from build123d import *

# Parameters (mm, degrees)
CROQUIS1_R              = 10
SALIENTE_EXTRUIR1_DEPTH = 5


with BuildPart() as part:
    # Croquis1 → Saliente-Extruir1 (new body, symmetric)
    with BuildSketch(Plane.XY):
        with BuildLine():
            Line((-55, 15), (55, 15))
            ThreePointArc((55, 15), (62.071067812, 12.071067812), (65, 5))
            Line((65, 5), (65, -5))
            ThreePointArc((65, -5), (62.071067812, -12.071067812), (55, -15))
            Line((55, -15), (-55, -15))
            ThreePointArc((-55, -15), (-62.071067812, -12.071067812), (-65, -5))
            Line((-65, -5), (-65, 5))
            ThreePointArc((-65, 5), (-62.071067812, 12.071067812), (-55, 15))
        make_face()
        with Locations((-50, 0)):
            Circle(CROQUIS1_R, mode=Mode.SUBTRACT)
        with Locations((50, 0)):
            Circle(CROQUIS1_R, mode=Mode.SUBTRACT)
    extrude(amount=SALIENTE_EXTRUIR1_DEPTH, both=True)


solid = part.part
Design review of the part built by this model. Coordinates are the model's own, in mm. Round coordinates to 2 decimals unless told otherwise and drop trailing zeros. Write each loop counter-clockwise with the first axis right and the second up, starting at its lowest first coordinate (ties: lowest second). Pieces come first, ordered by that corner, then holes. Notation, with made-up numbers: M -5.75,65.25 L 4.25,65.25 A26 cw 4.25,88.25 Z; hole C -31.5,-20 d7. An arc over 180 degrees is marked long. One line per item, written item: value. Start each with the question number.
1. Take a section at B-B on x = 50. State the section outline as (y, z) points.
2. Take a section at D-D on x = -50.5. State the section outline as (y, z) points.
3. Take a section at A-A on y = 0. State the section outline as (x, z) points, then the cut area to 3 significant figures.
4. Take a section at C-C on z = 0.75. State the section outline as (x, y) points, then the cut area to 3 significant figures.
5. Clearance check with a flat-ended pin moving along its axis: P1, Ø18, axis at x = -50, y = 0, coming from the -Z side. State where the tip first meets the part, or that it passes through.
6. To check wall thickness, follow probe 1 along X at (y, z) = (8.5, 0.25); probe 2 along Y at (x, z) = (-50, 2.25); probe 3 along X at (y, z) = (6, -2.25). State the ranges of each line that lie inside material, in increasing order. Write a range as from..to.
Computed:
1. outline: M -15,-5 L -10,-5 L -10,5 L -15,5 Z; M 10,-5 L 15,-5 L 15,5 L 10,5 Z
2. outline: M -15,-5 L -9.99,-5 L -9.99,5 L -15,5 Z; M 9.99,-5 L 15,-5 L 15,5 L 9.99,5 Z
3. outline: M -65,-5 L -60,-5 L -60,5 L -65,5 Z; M -40,-5 L 40,-5 L 40,5 L -40,5 Z; M 60,-5 L 65,-5 L 65,5 L 60,5 Z
3. area: 900 mm²
4. outline: M -65,-5 A10 ccw -55,-15 L 55,-15 A10 ccw 65,-5 L 65,5 A10 ccw 55,15 L -55,15 A10 ccw -65,5 Z; hole C -50,0 d20; hole C 50,0 d20
4. area: 3,190 mm²
5. P1: passes through
6. probe 1: x = -64.37..-55.27, -44.73..44.73, 55.27..64.37
6. probe 2: y = -15..-10, 10..15
6. probe 3: x = -64.95..-58, -42..42, 58..64.95
